from build123d import *

# Parameters (mm, degrees)
SKETCH_1_R          = 5.5
EXTRUDE_1_DEPTH     = 2.3
SKETCH_2_R          = 2
EXTRUDE_2_DEPTH     = 1.9
SKETCH_3_R          = 1
CUT_EXTRUDE_1_DEPTH = 9.839683252
SKETCH_4_R          = 4.75
CUT_EXTRUDE_2_DEPTH = 1.5


with BuildPart() as part:
    # 草图1 → 凸台-拉伸1 (new body)
    with BuildSketch(Plane(origin=(0, 0, 0), x_dir=(0, 0, -1), z_dir=(1, 0, 0))):
        Circle(SKETCH_1_R)
    extrude(amount=EXTRUDE_1_DEPTH)

    # 草图2 → 凸台-拉伸2 (add)
    with BuildSketch(Plane(origin=(2.3, 0, 0), x_dir=(0, 0, -1), z_dir=(1, 0, 0))):
        with Locations(Location((0, 0, 0), (0, 0, 180))):
            Circle(SKETCH_2_R)
    extrude(amount=EXTRUDE_2_DEPTH)

    # 草图3 → 切除-拉伸1 (cut, through all)
    with BuildSketch(Plane(origin=(4.2, 0, 0), x_dir=(0, 0, -1), z_dir=(1, 0, 0))):
        Circle(SKETCH_3_R)
    extrude(amount=-CUT_EXTRUDE_1_DEPTH, mode=Mode.SUBTRACT)

    # 草图4 → 切除-拉伸2 (cut)
    with BuildSketch(Plane.ZY):
        Circle(SKETCH_4_R)
    extrude(amount=-CUT_EXTRUDE_2_DEPTH, mode=Mode.SUBTRACT)


solid = part.part
For this review, take the finished solid that the model builds, in its own axes (mm). A direction names the side the tool comes from. Round coordinates to 2 decimals unless told otherwise and drop trailing zeros. Loops run counter-clockwise (first coordinate to the right, second up) from the corner with the lowest first, then second, coordinate; pieces in that order, holes last. Notation, with made-up numbers: (-22, 87) - (4, 87) arc R25 ccw to (4, 100) - close; hole circle Ø3 at (80, -4). An arc over 180 degrees is marked (long way). One line per item, written item: value. Start each with the question number.
Item 1: Take a section at A-A (z = 0). Give the boundary of the cut face in (x, y), plus the area to 4 significant figures.
Item 2: Take a section at C-C (x = 3.4). Give the boundary of the cut face in (y, z), plus the area to 3 significant figures.
Item 3: Take a section at D-D (y = 3.25). Give the boundary of the cut face in (x, z), plus the area to 3 significant figures.
Item 4: Clearance check with a flat-ended pin moving along its axis: pin 1 Ø3 at (y, z) = (0, 0) entering from -X. State where the tip first meets the part, or that it passes through.
Item 5: For faces 1 (the cylindrical face through (3, 2, 0)), 2 (the flat face through (1.5, -1, 1)), 3 (the flat face through (4.2, 1, 1)), list the 3-axis set-ups (+Z, -Z, +X, -X, +Y, -Y) from which the entire face can be reached by the end or side of a thin tool; tool diameter is ignored.
Item 6: The part is to be moulded in two halves that separate along Z. For faces 4 (the cylindrical face through (3, -1, 0)), 5 (the cylindrical face through (1.13, -5.37, 1.19)), 6 (the flat face through (2.3, -2.4, 0.1)), say which applies: +Z half, -Z half, draft (parallel to the pull), parting line (faces both ways), or undercut.
Item 7: For L1, parallel to Y at x = 1, z = 0; L2, parallel to Y at x = 2.15, z = 0; L3, parallel to X at y = -3, z = -0.25, list the stretches that pass through material, from the lowest coordinate up.
Answer below:
1. outline: (0, -5.5) - (2.3, -5.5) - (2.3, -2) - (4.2, -2) - (4.2, -1) - (1.5, -1) - (1.5, -4.75) - (0, -4.75) - close; (0, 4.75) - (1.5, 4.75) - (1.5, 1) - (4.2, 1) - (4.2, 2) - (2.3, 2) - (2.3, 5.5) - (0, 5.5) - close
1. area: 13.25 mm2
2. outline: circle Ø4 at (0, 0); hole circle Ø2 at (0, 0)
2. area: 9.42 mm2
3. outline: (0, -4.44) - (2.3, -4.44) - (2.3, 4.44) - (0, 4.44) - (0, 3.46) - (1.5, 3.46) - (1.5, -3.46) - (0, -3.46) - close
3. area: 10.0 mm2
4. pin 1: stops at x = 1.5
5. face 1: +X
5. face 2: -X
5. face 3: +Z, -Z, +X, +Y, -Y
6. face 4: undercut
6. face 5: parting line
6. face 6: draft
7. L1: y = -5.5 to -4.75, 4.75 to 5.5
7. L2: y = -5.5 to -1, 1 to 5.5
7. L3: x = 1.5 to 2.3
